The listing builds one solid part. Answer for the finished solid, in the listing's coordinates (mm). Face numbers are marked on the shaded views. A direction names the side the tool comes from. Coordinates: 2 decimals unless noted, no trailing zeros. Write each loop counter-clockwise with the first axis right and the second up, starting at its lowest first coordinate (ties: lowest second). Pieces come first, ordered by that corner, then holes.
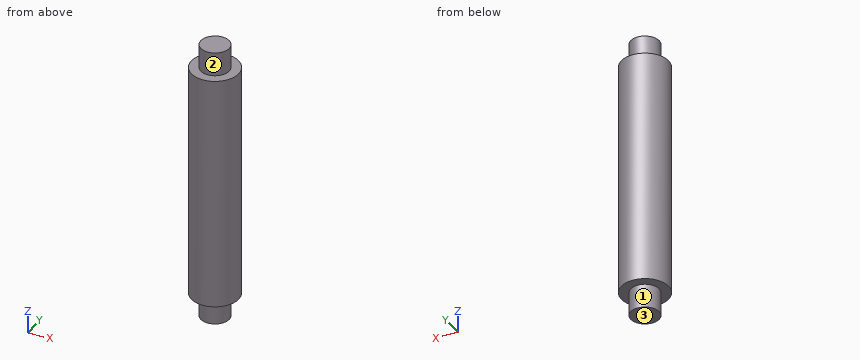
from build123d import *

# Parameters (mm, degrees)
F0_R     = 10
F1_DEPTH = 50
F2_R     = 6
F3_DEPTH = 10.1


with BuildPart() as f1:
    # F0 (on Top) → F1 (new body, symmetric)
    with BuildSketch(Plane.XY):
        Circle(F0_R)
    extrude(amount=F1_DEPTH, both=True)

    # F2 (on face) → F3 (join)
    with BuildSketch(Plane.XY.offset(50)):
        Circle(F2_R)
    extrude(amount=F3_DEPTH)

    # F4: F1 across plane


with BuildPart() as f1_1:
    add(f1.part)
    add(f1.part.mirror(Plane.XY))


solid = f1_1.part
1. Find the intervals of material crossed by L1, parallel to Z at x = -2.75, y = -8; L2, parallel to Y at x = -8, z = -38; L3, parallel to X at y = 5.25, z = -48, in increasing order.
Results found:
L1: z = -50 to 50
L2: y = -6 to 6
L3: x = -8.51 to 8.51
2. Section D-D on x = -8.25 is taken. Give the vertices of the cut face in (y, z).
Results found:
outline: (-5.65, -50) - (5.65, -50) - (5.65, 50) - (-5.65, 50) - close
3. Section C-C on z = 29 is taken. Give the vertices of the cut face in (x, y), then the cut area to 3 significant figures.
Results found:
outline: circle Ø20 at (0, 0)
area: 314 mm2
4. Flat-ended cylindrical pins translate along their axes: P1, Ø1.5, axis at x = -5.5, z = -45, coming from the +Y side; P2, Ø10, axis at x = -7.5, z = -16, coming from the +Y side; P3, Ø4, axis at y = 6, z = 18, coming from the +X side. Find the tip coordinate at first contact, or state that the pin passes through.
Results found:
P1: stops at y = 8.8
P2: stops at y = 9.68
P3: stops at x = 9.17
5. A tool of negligible diameter and unlimited length cuts with its end or side. For the marked faces 1, 2 and 3, from which of +Z, -Z, +X, -X, +Y, -Y can it reach the whole face along a straight path? Write none if from no direction.
Results found:
face 1: -Z
face 2: +Z
face 3: -Z, +X, -X, +Y, -Y
6. Section A-A on y = 0 is taken. Give the vertices of the cut face in (x, z), then the cut area to 3 significant figures.
Results found:
outline: (-10, -50) - (-6, -50) - (-6, -60.1) - (6, -60.1) - (6, -50) - (10, -50) - (10, 50) - (6, 50) - (6, 60.1) - (-6, 60.1) - (-6, 50) - (-10, 50) - close
area: 2,240 mm2
